Part model, mm, in its own coordinate system. A direction names the side the tool comes from. Coordinates: 2 decimals unless noted, no trailing zeros. Write each loop counter-clockwise with the first axis right and the second up, starting at its lowest first coordinate (ties: lowest second). Pieces come first, ordered by that corner, then holes. Notation, with made-up numbers: (-24, 73.25) -> (-13, 73.25) arc R21 ccw to (-13, 98.25) -> close; hole circle Ø3 at (67.25, 73). An arc over 180 degrees is marked (long way). Write item = value, one per line.
from build123d import *

# Parameters (mm, degrees)
SKETCH001_W     = 90.71
SKETCH001_H     = 53.7
PAD_DEPTH       = 2
SKETCH002_W     = 61.57
SKETCH002_H     = 44.62
POCKET_DEPTH    = 2.001
SKETCH004_W     = 90.71
SKETCH004_H     = 53.7
SKETCH004_W_2   = 61.57
SKETCH004_H_2   = 44.62
PAD001_DEPTH    = 9.25
POCKET001_DEPTH = 25.5
POCKET002_DEPTH = 1.351
FILLET_R        = 3
SKETCH006_R     = 2.2
HOLE_DEPTH      = 7
POCKET007_DEPTH = 6.5
FILLET002_R     = 2.5
FILLET003_R     = 1
SKETCH014_R     = 1.5
POCKET008_DEPTH = 2.25
FILLET004_R     = 1


with BuildPart() as part:
    # Sketch001 → Pad (new body)
    with BuildSketch(Plane.XY):
        with Locations((-2.23, 0)):
            Rectangle(SKETCH001_W, SKETCH001_H)
    extrude(amount=-PAD_DEPTH)

    # Sketch002 (on Face5 of Pad) → Pocket (cut, through all)
    with BuildSketch(Plane.XY):
        with Locations((-1.8, 0)):
            Rectangle(SKETCH002_W, SKETCH002_H)
    extrude(amount=-POCKET_DEPTH, mode=Mode.SUBTRACT)

    # Sketch004 (on Face5 of Pocket) → Pad001 (join)
    with BuildSketch(Plane(origin=(0, 0, -2), x_dir=(1, 0, 0), z_dir=(0, 0, -1))):
        with Locations((-2.23, 0)):
            Rectangle(SKETCH004_W, SKETCH004_H)
        with Locations((-1.8, 0)):
            Rectangle(SKETCH004_W_2, SKETCH004_H_2, mode=Mode.SUBTRACT)
    extrude(amount=PAD001_DEPTH)

    # Sketch003 → Pocket001 (cut, symmetric)
    with BuildSketch(Plane.XZ):
        Polygon((-34.5, -15.15), (-34.5, -10.15), (-35.5, -9.15), (-35.5, -2), (0, -2), (0, -15.15), align=None)
    pocket001 = extrude(amount=POCKET001_DEPTH, both=True, mode=Mode.SUBTRACT)

    # Mirrored: Pocket001 across YZ
    add(pocket001.mirror(Plane.YZ), mode=Mode.SUBTRACT)

    # Sketch005 (on Face20 of Mirrored) → Pocket002 (cut, through all)
    with BuildSketch(Plane.XZ.offset(-25.5)):
        Polygon((-34.5, -11.25), (-34.5, -10.15), (-35.5, -9.15), (-35.5, -2), (35.5, -2), (35.5, -9.15), (34.5, -10.15), (34.5, -11.25), align=None)
    extrude(amount=-POCKET002_DEPTH, mode=Mode.SUBTRACT)

    # Fillet
    fillet_edges = [part.edges().sort_by_distance(p)[0] for p in [
        (43.125, 26.85, -1),
        (43.125, 26.85, -6.625),
        (43.125, -26.85, -1),
        (43.125, -26.85, -6.625),
        (-47.585, -26.85, -1),
        (-47.585, -26.85, -6.625),
        (-47.585, 26.85, -1),
        (-47.585, 26.85, -6.625),
    ]]
    fillet(fillet_edges, radius=FILLET_R)

    # Sketch006 (on Face17 of Fillet) → Hole (cut)
    with BuildSketch(Plane(origin=(0, 0, -11.25), x_dir=(1, 0, 0), z_dir=(0, 0, -1))):
        with Locations((-43.585, 22.85)):
            Circle(SKETCH006_R)
        with Locations((-43.585, -22.85)):
            Circle(SKETCH006_R)
        with Locations((39.125, -22.85)):
            Circle(SKETCH006_R)
        with Locations((39.125, 22.85)):
            Circle(SKETCH006_R)
        with Locations((-43.585, 22.85)):
            Circle(SKETCH006_R)
        with Locations((-43.585, -22.85)):
            Circle(SKETCH006_R)
        with Locations((39.125, 22.85)):
            Circle(SKETCH006_R)
        with Locations((39.125, -22.85)):
            Circle(SKETCH006_R)
    extrude(amount=-HOLE_DEPTH, mode=Mode.SUBTRACT)

    # Sketch011 → Pocket007 (cut, symmetric)
    with BuildSketch(Plane.XZ):
        Polygon((-37.085, 0), (-37.085, -11.25), (-47.585, -11.25), (-47.585, -6.75), (-41.585, -6.75), (-41.585, 0), align=None)
    extrude(amount=POCKET007_DEPTH, both=True, mode=Mode.SUBTRACT)

    # Fillet002
    fillet002_edges = [part.edges().sort_by_distance(p)[0] for p in [
        (-41.585, 0, -6.75),
    ]]
    fillet(fillet002_edges, radius=FILLET002_R)

    # Fillet003
    fillet003_edges = [part.edges().sort_by_distance(p)[0] for p in [
        (-41.585, -6.5, -2.125),
        (-37.085, -6.5, -5.625),
        (-37.085, 6.5, -5.625),
        (-41.585, 6.5, -2.125),
    ]]
    fillet(fillet003_edges, radius=FILLET003_R)

    # Sketch014 (on Face4 of Fillet003) → Pocket008 (cut)
    with BuildSketch(Plane(origin=(0, 0, -11.25), x_dir=(1, 0, 0), z_dir=(0, 0, -1))):
        with Locations((-42.585, 16)):
            Circle(SKETCH014_R)
        with Locations((-42.585, -16)):
            Circle(SKETCH014_R)
    extrude(amount=-POCKET008_DEPTH, mode=Mode.SUBTRACT)

    # Fillet004
    fillet004_edges = [part.edges().sort_by_distance(p)[0] for p in [
        (-44.085, -16, -9),
        (-44.085, 16, -9),
    ]]
    fillet(fillet004_edges, radius=FILLET004_R)


solid = part.part
Q1. Pin check, flat tips, straight feed: pin 1 (2 mm diameter, centred on x = -44, y = 22.5, fed in from -Z); pin 2 (10 mm diameter, centred on x = -28, y = 20, fed in from -Z). Stop position of each tip, or through.
Model answer:
pin_1 = -4.25
pin_2 = -2
Q2. Probe line 1 (X direction, y = 1, z = -3.5) (3 decimals); line 2 (X direction, y = 16, z = -10.6) (3 decimals); line 3 (X direction, y = -22.85, z = -7.5) (3 decimals). List the from-to ranges inside material, lowest first. Write a range as from..to.
Model answer:
line_1 = -47.585..-41.585, -37.085..-35.5, 35.5..43.125
line_2 = -47.585..-44.085, -41.085..-34.5, 34.5..43.125
line_3 = -47.585..-45.785, -41.385..-35.5, 35.5..36.925, 41.325..43.125
Q3. Saw through at B-B on x = -10. Give the cut face in (y, z).
Model answer:
outline = (-26.85, -11.25) -> (-25.5, -11.25) -> (-25.5, -2) -> (-22.31, -2) -> (-22.31, 0) -> (-26.85, 0) -> close; (22.31, -2) -> (26.85, -2) -> (26.85, 0) -> (22.31, 0) -> close
Q4. Mould opens along Y. For faces 4 (the face through (-44.084, -16.066, -10.634)), 5 (the face through (-46.73, 25.95, -5.7)), 6 (the face through (35.5, 0, -6)) say: released by +Y, released by -Y, zero draft, split by the parting line, or undercut.
Model answer:
face_4 = undercut
face_5 = released by +Y
face_6 = zero draft
Q5. Which spindle directions (+Z, -Z, +X, -X, +Y, -Y) get a long thin tool onto all of the face, cutting with end or side? Do faces 1 (the face through (-32.585, 0, -1)), 2 (the face through (-44.084, 15.934, -10.634)), 3 (the face through (-47.585, 0, -6)). Say none if no direction does.
Model answer:
face_1 = +Z, -Z
face_2 = -Z
face_3 = +Z, -Z, -X, +Y, -Y
Q6. Saw through at A-A on y = 18.5. Give the cut face in (x, z) (3 decimals).
Model answer:
outline = (-47.585, -11.25) -> (-34.5, -11.25) -> (-34.5, -10.15) -> (-35.5, -9.15) -> (-35.5, -2) -> (-32.585, -2) -> (-32.585, 0) -> (-47.585, 0) -> close; (28.985, -2) -> (35.5, -2) -> (35.5, -9.15) -> (34.5, -10.15) -> (34.5, -11.25) -> (43.125, -11.25) -> (43.125, 0) -> (28.985, 0) -> close
